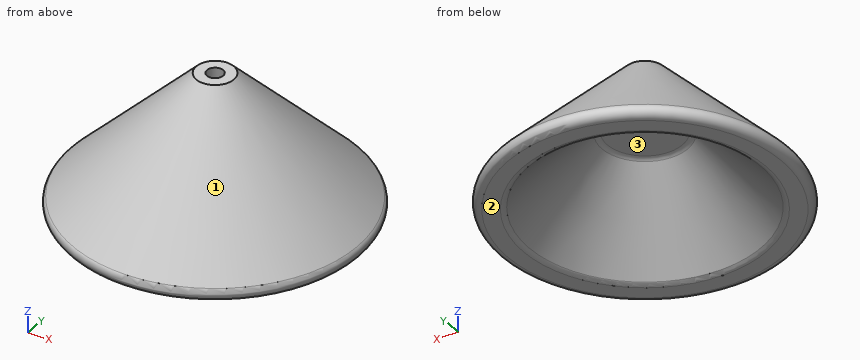
```python
from build123d import *

# Parameters (mm, degrees)
F3_D     = 5.5
F3_DEPTH = 12.7
F3_TIP   = 1.6523667023


with BuildPart() as f1:
    # F0 (on Front) → F1 (revolve)
    with BuildSketch(Plane.XZ):
        with BuildLine():
            Line((0, 46.0489243269), (0, 26.1994621634))
            Line((0, 26.1994621634), (12.7, 26.1994621634))
            ThreePointArc((12.7, 26.1994621634), (13.6720159182, 26.006116176), (14.4960512242, 25.4555133877))
            Line((14.4960512242, 25.4555133877), (39.2076158361, 0.7439487758))
            ThreePointArc((39.2076158361, 0.7439487758), (40.0316511421, 0.1933459874), (41.0036670603, 0))
            Line((41.0036670603, 0), (46.2668218785, 0))
            ThreePointArc((46.2668218785, 0), (48.613475891, 1.5679840818), (48.0628731027, 4.3360512242))
            Line((48.0628731027, 4.3360512242), (6.35, 46.0489243269))
            Line((6.35, 46.0489243269), (0, 46.0489243269))
        make_face()
    revolve(axis=Axis((0, 0, 36.1241932452), (0, 0, 1)))

    # F3
    with Locations(Plane.XY.offset(46.0489243269)):
        with Locations((0, 0)):
            Hole(F3_D / 2, depth=F3_DEPTH)
            with Locations((0, 0, -(F3_DEPTH + F3_TIP / 2))):  # 118° drill point
                Cone(0, F3_D / 2, F3_TIP, mode=Mode.SUBTRACT)


solid = f1.part
```
Can you work these out from the model? Positions are in its coordinate system, mm. Face numbers are marked on the shaded views. Give positions to 0.01 mm unless a question says otherwise; leave off trailing zeros. Order: outer loops, then holes, each group sorted by start corner. A loop starts at its lowest first (then second) coordinate and runs counter-clockwise, first axis right, second up. Notation, with made-up numbers: (-13, -34.5) - (18, -34.5) arc R18 ccw to (18, -21.5) - close; hole circle Ø5 at (38.5, -31.75). An arc over 180 degrees is marked (long way). Use a Markdown table: item, result. Add a question column.
Q1. If we mould it in two halves opening along X, with no side actions, what happens to the marked faces 1, 2 and 3? For each: released by +X, released by -X, zero draft, split by the parting line, or undercut.
Q2. If we section it at A-A on z = 18: Write out the boundary of the cut face in (x, y).
Q3. If we section it at B-B on z = 12.5: Write out the boundary of the cut face in (x, y).
Q4. Please list where these lines run through material, in increasing order: line 1 along X through (y, z) = (0, 40); line 2 along X through (y, z) = (0, 38.5); line 3 along Y through (x, z) = (0, 41.25).
Q5. I'm going to push flat-ended pins straight in: pin 1 (10 mm diameter, centred on x = 2.5, y = -14, fed in from -Z); pin 2 (2 mm diameter, centred on x = -4.5, y = -26.5, fed in from +Z); pin 3 (8 mm diameter, centred on y = -15.5, z = 12.5, fed in from -X). Where does each tip first touch, or does it pass through?
Answers follow:
| question | item | result |
|---|---|---|
| 1 | face 1 | split by the parting line |
| 1 | face 2 | zero draft |
| 1 | face 3 | undercut |
| 2 | outline | circle Ø68.8 at (0, 0); hole circle Ø43.9 at (0, 0) |
| 3 | outline | circle Ø79.8 at (0, 0); hole circle Ø54.9 at (0, 0) |
| 4 | line 1 | x = -12.4 to -2.75, 2.75 to 12.4 |
| 4 | line 2 | x = -13.9 to -2.75, 2.75 to 13.9 |
| 4 | line 3 | y = -11.15 to -2.75, 2.75 to 11.15 |
| 5 | pin 1 | stops at z = 20.73 |
| 5 | pin 2 | stops at z = 26.52 |
| 5 | pin 3 | stops at x = -41.31 |
